Check sheet for the modelled part. Datum: model origin and axes. Units: mm. Face numbers are marked on the shaded views. Round coordinates to 2 decimals unless told otherwise and drop trailing zeros. Write each loop counter-clockwise with the first axis right and the second up, starting at its lowest first coordinate (ties: lowest second). Pieces come first, ordered by that corner, then holes.
Item 1: Section check A-A, the plane z = 0. Record the cut outline in (x, y).
Item 2: Section check B-B, the plane y = 9.5. Record the cut outline in (x, z).
Item 3: Material ranges on line 1 along X through (y, z) = (1.6, 0); line 2 along X through (y, z) = (1.2, 18); line 3 along Z through (x, y) = (-26.5, 4), recorded low to high.
Item 4: Section check C-C, the plane x = -19. State how many separate pieces and enclosed holes the cut face has, plus the area to 3 significant figures.
Item 5: Release check for a two-part mould opening along Z. For the marked faces 1, 2 and 3 record: pulls with the +Z half, pulls with the -Z half, needs draft (parallel to the pull), parting line crosses it, or undercut.
Item 6: Depth check by flat-ended pin: pin 1 (1 mm diameter, centred on x = -24.5, z = -6, fed in from +Y); pin 2 (2.5 mm diameter, centred on x = -18, z = 18, fed in from +Y); pin 3 (1 mm diameter, centred on x = -27.5, y = 8.5, fed in from -Z); pin 4 (5 mm diameter, centred on x = -8.5, y = 7.5, fed in from +Z). Enter the tip coordinate at first touch or a pass-through.
from build123d import *

# Parameters (mm, degrees)
SKETCH_1_R          = 35
SKETCH_1_R_2        = 8
EXTRUDE_1_DEPTH     = 3
SKETCH_2_R          = 35
SKETCH_2_R_2        = 2
EXTRUDE_2_DEPTH     = 9
SKETCH_3_R          = 1.5
CUT_EXTRUDE_1_DEPTH = 8
SKETCH_4_R          = 2.50640253
CUT_EXTRUDE_2_DEPTH = 8
SKETCH_7_R          = 2
CUT_EXTRUDE_4_DEPTH = 12
EXTRUDE_4_DEPTH     = 1
SKETCH_9_W          = 15.497656666
SKETCH_9_H          = 9.48184561
CUT_EXTRUDE_5_DEPTH = 11
CHAMFER_1_SIZE      = 0.4


with BuildPart() as part:
    # Эскиз1 → Бобышка-Вытянуть1 (new body)
    with BuildSketch(Plane(origin=(0, 0, 0), x_dir=(1, 0, 0), z_dir=(0, 1, 0))):
        with Locations(Location((0, 0, 0), (0, 0, 270))):
            Circle(SKETCH_1_R)
        with Locations(Location((0, 0, 0), (0, 0, 270))):
            Circle(SKETCH_1_R_2, mode=Mode.SUBTRACT)
    extrude(amount=EXTRUDE_1_DEPTH)

    # Эскиз2 → Бобышка-Вытянуть2 (add)
    with BuildSketch(Plane(origin=(0, 3, 0), x_dir=(1, 0, 0), z_dir=(0, 1, 0))):
        with Locations(Location((0, 0, 0), (0, 0, 270))):
            Circle(SKETCH_2_R)
        with Locations(Location((-0.113661048, 30, 0), (0, 0, 270))):
            Circle(SKETCH_2_R_2, mode=Mode.SUBTRACT)
        with Locations(Location((26.037592637, -14.901566645, 0), (0, 0, 270))):
            Circle(SKETCH_2_R_2, mode=Mode.SUBTRACT)
        with Locations(Location((-25.92393159, -15.098433355, 0), (0, 0, 270))):
            Circle(SKETCH_2_R_2, mode=Mode.SUBTRACT)
        with BuildLine():
            ThreePointArc((-8.117111797, 30.953392319), (-27.773232815, 15.894890343), (-30.80008796, -8.680701679))
            ThreePointArc((-30.80008796, -8.680701679), (-29.387206086, -10.479447295), (-27.117120464, -10.75950488))
            ThreePointArc((-27.117120464, -10.75950488), (-22.03536976, -12.833684606), (-22.738725961, -18.277185484))
            ThreePointArc((-22.738725961, -18.277185484), (-23.615248532, -20.389868414), (-22.747868184, -22.506321181))
            ThreePointArc((-22.747868184, -22.506321181), (0.121237581, -31.999770334), (22.917752157, -22.333307773))
            ThreePointArc((22.917752157, -22.333307773), (23.769070618, -20.210343369), (22.87656479, -18.10436276))
            ThreePointArc((22.87656479, -18.10436276), (22.131981773, -12.666347691), (27.197869919, -10.55372159))
            ThreePointArc((27.197869919, -10.55372159), (29.465768293, -10.256470938), (30.86497998, -8.447071138))
            ThreePointArc((30.86497998, -8.447071138), (27.651995235, 16.104879992), (7.882335804, 31.014009452))
            ThreePointArc((7.882335804, 31.014009452), (5.618135468, 30.689790665), (4.240555674, 28.863867639))
            ThreePointArc((4.240555674, 28.863867639), (-0.096612013, 25.500032297), (-4.459143958, 28.830907074))
            ThreePointArc((-4.459143958, 28.830907074), (-5.850519761, 30.646339352), (-8.117111797, 30.953392319))
        make_face(mode=Mode.SUBTRACT)
    extrude(amount=EXTRUDE_2_DEPTH)

    # Эскиз3 → Вырез-Вытянуть1 (cut)
    with BuildSketch(Plane(origin=(0, 3, 0), x_dir=(1, 0, 0), z_dir=(0, 1, 0))):
        with Locations(Location((22.8, 0, 0), (0, 0, 270))):
            Circle(SKETCH_3_R)
        with Locations(Location((-22.8, 0, 0), (0, 0, 270))):
            Circle(SKETCH_3_R)
    extrude(amount=-CUT_EXTRUDE_1_DEPTH, mode=Mode.SUBTRACT)

    # Эскиз4 → Вырез-Вытянуть2 (cut)
    with BuildSketch(Plane(origin=(0, 3, 0), x_dir=(1, 0, 0), z_dir=(0, 1, 0))):
        with Locations(Location((0, 18, 0), (0, 0, 270))):
            Circle(SKETCH_4_R)
        with Locations(Location((15.588457268, -9, 0), (0, 0, 270))):
            Circle(SKETCH_4_R)
        with Locations(Location((-15.588457268, -9, 0), (0, 0, 270))):
            Circle(SKETCH_4_R)
    extrude(amount=-CUT_EXTRUDE_2_DEPTH, mode=Mode.SUBTRACT)

    # Эскиз7 → Вырез-Вытянуть4 (cut)
    with BuildSketch(Plane(origin=(0, 3, 0), x_dir=(1, 0, 0), z_dir=(0, 1, 0))):
        with Locations(Location((-18, -18, 0), (0, 0, 270))):
            Circle(SKETCH_7_R)
        with Locations(Location((18, -18, 0), (0, 0, 270))):
            Circle(SKETCH_7_R)
        with Locations(Location((-18, 18, 0), (0, 0, 270))):
            Circle(SKETCH_7_R)
        with Locations(Location((18, 18, 0), (0, 0, 270))):
            Circle(SKETCH_7_R)
    extrude(amount=-CUT_EXTRUDE_4_DEPTH, mode=Mode.SUBTRACT)

    # Эскиз8 → Бобышка-Вытянуть4 (add)
    with BuildSketch(Plane(origin=(0, 3, 0), x_dir=(1, 0, 0), z_dir=(0, 1, 0))):
        with BuildLine():
            Line((-13.748828333, -28.895842598), (13.748828333, -28.895842598))
            ThreePointArc((13.748828333, -28.895842598), (0, -32), (-13.748828333, -28.895842598))
        make_face()
    extrude(amount=EXTRUDE_4_DEPTH)

    # Эскиз9 → Вырез-Вытянуть5 (cut)
    with BuildSketch(Plane(origin=(0, 0, 28.895842598), x_dir=(-1, 0, 0), z_dir=(0, 0, -1))):
        with Locations((0, 8.740922805)):
            Rectangle(SKETCH_9_W, SKETCH_9_H)
    extrude(amount=-CUT_EXTRUDE_5_DEPTH, mode=Mode.SUBTRACT)

    # Фаска1
    chamfer_1_edges = [part.edges().sort_by_distance(p)[0] for p in [
        (15.940347108, 12, 27.747168037),
        (7.748828333, 12, 32.589541055),
        (-7.748828333, 12, 32.589541055),
        (0, 12, -35),
        (-29.387206086, 12, 10.479447295),
        (-22.03536976, 12, 12.833684606),
        (-23.615248532, 12, 20.389868414),
        (-15.835107718, 12, 27.807361679),
        (23.769070618, 12, 20.210343369),
        (22.131981773, 12, 12.666347691),
        (29.465768293, 12, 10.256470938),
        (27.651995235, 12, -16.104879992),
        (5.618135468, 12, -30.689790665),
        (-0.096612013, 12, -25.500032297),
        (-5.850519761, 12, -30.646339352),
        (-27.773232815, 12, -15.894890343),
        (-0.113661048, 12, -32),
        (26.037592637, 12, 12.901566645),
        (-25.92393159, 12, 13.098433355),
    ]]
    chamfer(chamfer_1_edges, length=CHAMFER_1_SIZE)


solid = part.part
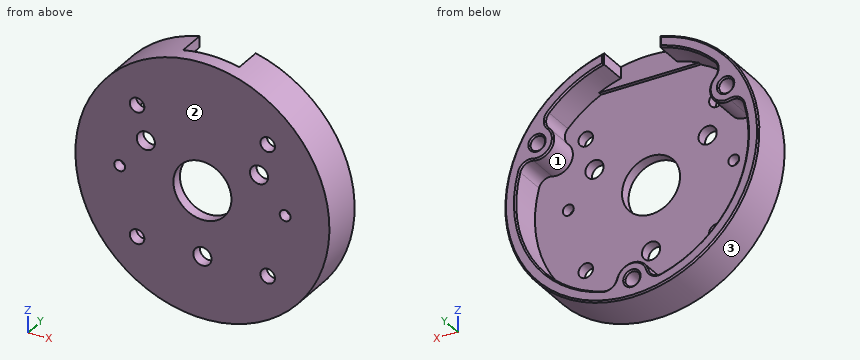
Values found:
1. outline: (-35, 0) - (-24.3, 0) - (-24.3, 3) - (-32, 3) - (-32, 11.6) - (-32.4, 12) - (-34.6, 12) - (-35, 11.6) - close; (-21.3, 0) - (-8, 0) - (-8, 3) - (-21.3, 3) - close; (8, 0) - (21.3, 0) - (21.3, 3) - (8, 3) - close; (24.3, 0) - (35, 0) - (35, 11.6) - (34.6, 12) - (32.4, 12) - (32, 11.6) - (32, 3) - (24.3, 3) - close
2. outline: (-30.8, 8.68) arc R3 cw to (-27.12, 10.76) arc R4.5 ccw to (-22.74, 18.28) arc R3 cw to (-22.75, 22.51) arc R32 cw to (-7.75, 31.05) - (-7.75, 34.13) arc R35 ccw (long way) to (7.75, 34.13) - (7.75, 31.05) arc R32 cw to (22.92, 22.33) arc R3 cw to (22.88, 18.1) arc R4.5 ccw to (27.2, 10.55) arc R3 cw to (30.86, 8.45) arc R32 cw to (7.88, -31.01) arc R3 cw to (4.24, -28.86) arc R4.5 ccw to (-4.46, -28.83) arc R3 cw to (-8.12, -30.95) arc R32 cw to start; hole circle Ø4 at (-25.92, 15.1); hole circle Ø4 at (-0.11, -30); hole circle Ø4 at (26.04, 14.9)
3. line 1: x = -35 to -24.3, -21.3 to -8, 8 to 21.3, 24.3 to 35
3. line 2: x = -30.02 to -20, -16 to 16, 20 to 30.02
3. line 3: z = -22.86 to -17.94, 10.64 to 13.18, 17.01 to 22.86
4. separate pieces: 3
4. enclosed holes: 0
4. area: 221 mm2
5. face 1: undercut
5. face 2: needs draft
5. face 3: parting line crosses it
6. pin 1: stops at y = 3
6. pin 2: passes through
6. pin 3: stops at z = -22.27
6. pin 4: stops at z = 34.13
